Check sheet for the modelled part. Datum: model origin and axes. Units: mm. Round coordinates to 2 decimals unless told otherwise and drop trailing zeros. Order: outer loops, then holes, each group sorted by start corner. A loop starts at its lowest first (then second) coordinate and runs counter-clockwise, first axis right, second up. Notation, with made-up numbers: (35, 18) -> (75, 18) arc R23 ccw to (75, 47) -> close; hole circle Ø2 at (-32, 78). An arc over 180 degrees is marked (long way). Answer in a Markdown table with one row per item.
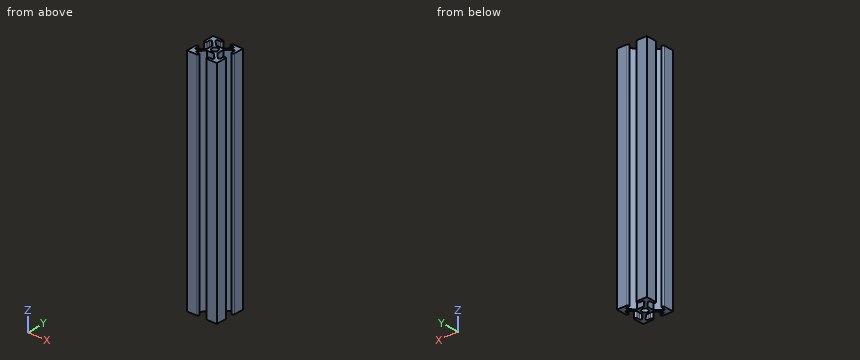
```python
from build123d import *

# Parameters (mm, degrees)
SKETCH1_R           = 2.6035
BOSS_EXTRUDE1_DEPTH = 190.5


with BuildPart() as part:
    # Sketch1 → Boss-Extrude1 (new body)
    with BuildSketch(Plane.XY):
        with BuildLine():
            Line((-12.7, -12.7), (-4.343399971, -12.7))
            ThreePointArc((-4.343399971, -12.7), (-3.238499971, -11.5951), (-4.343399971, -10.4902))
            Line((-4.343399971, -10.4902), (-6.474794456, -10.4902))
            ThreePointArc((-6.474794456, -10.4902), (-7.413456061, -9.863006367), (-7.193214945, -8.75577951))
            Line((-7.193214945, -8.75577951), (-2.933235435, -4.4958))
            Line((-2.933235435, -4.4958), (2.933235435, -4.4958))
            Line((2.933235435, -4.4958), (7.193214945, -8.75577951))
            ThreePointArc((7.193214945, -8.75577951), (7.413456061, -9.863006367), (6.474794456, -10.4902))
            Line((6.474794456, -10.4902), (4.3434, -10.4902))
            ThreePointArc((4.3434, -10.4902), (3.2385, -11.5951), (4.3434, -12.7))
            Line((4.3434, -12.7), (12.7, -12.7))
            Line((12.7, -12.7), (12.7, -4.343399971))
            ThreePointArc((12.7, -4.343399971), (11.5951, -3.238499971), (10.4902, -4.343399971))
            Line((10.4902, -4.343399971), (10.4902, -6.474794456))
            ThreePointArc((10.4902, -6.474794456), (9.863006367, -7.413456061), (8.75577951, -7.193214945))
            Line((8.75577951, -7.193214945), (4.4958, -2.933235435))
            Line((4.4958, -2.933235435), (4.4958, 2.933235435))
            Line((4.4958, 2.933235435), (8.75577951, 7.193214945))
            ThreePointArc((8.75577951, 7.193214945), (9.863006367, 7.413456061), (10.4902, 6.474794456))
            Line((10.4902, 6.474794456), (10.4902, 4.3434))
            ThreePointArc((10.4902, 4.3434), (11.5951, 3.2385), (12.7, 4.3434))
            Line((12.7, 4.3434), (12.7, 12.7))
            Line((12.7, 12.7), (4.343399971, 12.7))
            ThreePointArc((4.343399971, 12.7), (3.238499971, 11.5951), (4.343399971, 10.4902))
            Line((4.343399971, 10.4902), (6.474794456, 10.4902))
            ThreePointArc((6.474794456, 10.4902), (7.413456061, 9.863006367), (7.193214945, 8.75577951))
            Line((7.193214945, 8.75577951), (2.933235435, 4.4958))
            Line((2.933235435, 4.4958), (-2.933235435, 4.4958))
            Line((-2.933235435, 4.4958), (-7.193214945, 8.75577951))
            ThreePointArc((-7.193214945, 8.75577951), (-7.413456061, 9.863006367), (-6.474794456, 10.4902))
            Line((-6.474794456, 10.4902), (-4.3434, 10.4902))
            ThreePointArc((-4.3434, 10.4902), (-3.2385, 11.5951), (-4.3434, 12.7))
            Line((-4.3434, 12.7), (-12.7, 12.7))
            Line((-12.7, 12.7), (-12.7, 4.343399971))
            ThreePointArc((-12.7, 4.343399971), (-11.5951, 3.238499971), (-10.4902, 4.343399971))
            Line((-10.4902, 4.343399971), (-10.4902, 6.474794456))
            ThreePointArc((-10.4902, 6.474794456), (-9.863006367, 7.413456061), (-8.75577951, 7.193214945))
            Line((-8.75577951, 7.193214945), (-4.4958, 2.933235435))
            Line((-4.4958, 2.933235435), (-4.4958, -2.933235435))
            Line((-4.4958, -2.933235435), (-8.75577951, -7.193214945))
            ThreePointArc((-8.75577951, -7.193214945), (-9.863006367, -7.413456061), (-10.4902, -6.474794456))
            Line((-10.4902, -6.474794456), (-10.4902, -4.3434))
            ThreePointArc((-10.4902, -4.3434), (-11.5951, -3.2385), (-12.7, -4.3434))
            Line((-12.7, -4.3434), (-12.7, -12.7))
        make_face()
        with Locations(Location((0, 0, 0), (0, 0, 180))):
            Circle(SKETCH1_R, mode=Mode.SUBTRACT)
    extrude(amount=-BOSS_EXTRUDE1_DEPTH)


solid = part.part
```
(1) Section check A-A on y = 0. Record the boundary of the cut face in (x, z).
Solutions:
| item | result |
|---|---|
| outline | (-4.5, -190.5) -> (-2.6, -190.5) -> (-2.6, 0) -> (-4.5, 0) -> close; (2.6, -190.5) -> (4.5, -190.5) -> (4.5, 0) -> (2.6, 0) -> close |
(2) Scan lines: probe 1 along X at (y, z) = (-0.25, -89); probe 2 along Y at (x, z) = (0, -117); probe 3 along X at (y, z) = (-7.25, -20). Record each from-to range of solid material in increasing order. Write a range as from..to.
Solutions:
| item | result |
|---|---|
| probe 1 | -4.5..-2.59, 2.59..4.5 |
| probe 2 | -4.5..-2.6, 2.6..4.5 |
| probe 3 | -12.7..-10.13, -8.82..-5.69, 5.69..8.82, 10.13..12.7 |
(3) Depth check by flat-ended pin: pin 1 Ø5 at (y, z) = (-0.5, -156.5) entering from +X; pin 2 Ø3 at (x, y) = (0, 0) entering from +Z; pin 3 Ø4.5 at (x, z) = (0.5, -112.5) entering from -Y; pin 4 Ø6.5 at (x, z) = (-0.5, -104.5) entering from +Y. Enter the tip coordinate at first touch or a pass-through.
Solutions:
| item | result |
|---|---|
| pin 1 | x = 4.56 |
| pin 2 | through |
| pin 3 | y = -4.5 |
| pin 4 | y = 12.53 |
